```python
from build123d import *

# Parameters (mm, degrees)
F1_DEPTH  = 3.3
F0_W      = 178
F0_H      = 101.8
F2_DEPTH  = 2.5
F3_W      = 142.8
F3_H      = 4
F4_DEPTH  = 4
F5_R      = 1.99999
F7_D      = 2
F3_W_2    = 26.3
F8_DEPTH  = 0.1
F10_DEPTH = 0.5
F3_W_3    = 2.5
F3_H_2    = 8
F11_DEPTH = 10
F12_R     = 3.99999
F13_R     = 2
F14_DEPTH = 10


# Not quite as in the source:
# - a fillet or chamfer is up to 0.001 mm smaller than in the source, because OpenCascade refuses the exact size


with BuildPart() as f1:
    # F0 (on Front) → F1 (new body)
    with BuildSketch(Plane.XZ):
        with BuildLine():
            ThreePointArc((-75.5207621713, 74.1601898761), (-81.9271496089, 71.5065773137), (-84.5807621713, 65.1001898761))
            Line((-84.5807621713, 65.1001898761), (-84.5807621713, -35.3734344864))
            Line((-84.5807621713, -35.3734344864), (-84.5807621713, -55.8398101239))
            Line((-84.5807621713, -55.8398101239), (110.8192378287, -55.8398101239))
            Line((110.8192378287, -55.8398101239), (110.8192378287, -35.3734344864))
            Line((110.8192378287, -35.3734344864), (110.8192378287, 65.1001898761))
            ThreePointArc((110.8192378287, 65.1001898761), (108.1656252662, 71.5065773137), (101.7592378287, 74.1601898761))
            Line((101.7592378287, 74.1601898761), (-75.5207621713, 74.1601898761))
        make_face()
        with BuildLine():
            ThreePointArc((-83.3807621713, 65.1001898761), (-81.0786214714, 70.6580491763), (-75.5207621713, 72.9601898761))
            Line((-75.5207621713, 72.9601898761), (101.7592378287, 72.9601898761))
            ThreePointArc((101.7592378287, 72.9601898761), (107.3170971288, 70.6580491763), (109.6192378287, 65.1001898761))
            Line((109.6192378287, 65.1001898761), (109.6192378287, -29.9798101239))
            ThreePointArc((109.6192378287, -29.9798101239), (107.3170971288, -35.537669424), (101.7592378287, -37.8398101239))
            Line((101.7592378287, -37.8398101239), (-75.5207621713, -37.8398101239))
            ThreePointArc((-75.5207621713, -37.8398101239), (-81.0786214714, -35.537669424), (-83.3807621713, -29.9798101239))
            Line((-83.3807621713, -29.9798101239), (-83.3807621713, 65.1001898761))
        make_face(mode=Mode.SUBTRACT)
    extrude(amount=F1_DEPTH)

    # F0 (on Front) → F2 (join)
    with BuildSketch(Plane.XZ):
        with BuildLine():
            Line((101.7592378287, 72.9601898761), (-75.5207621713, 72.9601898761))
            ThreePointArc((-75.5207621713, 72.9601898761), (-81.0786214714, 70.6580491763), (-83.3807621713, 65.1001898761))
            Line((-83.3807621713, 65.1001898761), (-83.3807621713, -29.9798101239))
            ThreePointArc((-83.3807621713, -29.9798101239), (-81.0786214714, -35.537669424), (-75.5207621713, -37.8398101239))
            Line((-75.5207621713, -37.8398101239), (101.7592378287, -37.8398101239))
            ThreePointArc((101.7592378287, -37.8398101239), (107.3170971288, -35.537669424), (109.6192378287, -29.9798101239))
            Line((109.6192378287, -29.9798101239), (109.6192378287, 65.1001898761))
            ThreePointArc((109.6192378287, 65.1001898761), (107.3170971288, 70.6580491763), (101.7592378287, 72.9601898761))
        make_face()
        with Locations((9.6192378287, 16.0601898761)):
            Rectangle(F0_W, F0_H, mode=Mode.SUBTRACT)
    extrude(amount=F2_DEPTH)

    # F3 (on face) → F4 (join)
    with BuildSketch(Plane(origin=(0, 0, 0), x_dir=(-1, 0, 0), z_dir=(0, 1, 0))):
        with Locations((-13.1192378287, -53.8398101239)):
            Rectangle(F3_W, F3_H)
    extrude(amount=F4_DEPTH)

    # F5 (radius 2 in the source; OpenCascade refuses exactly that, so slightly less here)
    f5_edges = [f1.edges().sort_by_distance(p)[0] for p in [
        (13.119238, 4, -51.83981),
        (13.119238, 4, -55.83981),
    ]]
    fillet(f5_edges, radius=F5_R)

    # F7 (through all)
    with Locations(Plane.YZ.offset(84.5192378287)):
        with Locations((2, -53.8398101239)):
            Hole(F7_D / 2)

    # F3 (on face) → F8 (cut)
    with BuildSketch(Plane(origin=(0, 0, 0), x_dir=(-1, 0, 0), z_dir=(0, 1, 0))):
        with Locations((-97.6692378287, -53.8398101239)):
            Rectangle(F3_W_2, F3_H)
        with Locations((71.4307621713, -53.8398101239)):
            Rectangle(F3_W_2, F3_H)
    extrude(amount=-F8_DEPTH, mode=Mode.SUBTRACT)

    # F9 (on face) → F10 (join)
    with BuildSketch(Plane.XZ.offset(3.3)):
        with BuildLine():
            Line((101.7592378287, 74.1601898761), (-75.5207621713, 74.1601898761))
            ThreePointArc((-75.5207621713, 74.1601898761), (-81.9271496089, 71.5065773137), (-84.5807621713, 65.1001898761))
            Line((-84.5807621713, 65.1001898761), (-84.5807621713, -55.8398101239))
            Line((-84.5807621713, -55.8398101239), (110.8192378287, -55.8398101239))
            Line((110.8192378287, -55.8398101239), (110.8192378287, 65.1001898761))
            ThreePointArc((110.8192378287, 65.1001898761), (108.1656252662, 71.5065773137), (101.7592378287, 74.1601898761))
        make_face()
        with BuildLine():
            add(Edge.make_bspline(
                [(14.902347951, -49.9172276662), (15.0190761779, -50.0441554468), (15.2457329289, -50.0441554468)],
                knots=[0, 0, 0, 1, 1, 1], degree=2))
            add(Edge.make_bspline(
                [(15.2457329289, -50.0441554468), (15.5585192454, -50.0441554468), (15.8418401843, -49.9308270713)],
                knots=[0, 0, 0, 1, 1, 1], degree=2))
            Line((15.8418401843, -49.9308270713), (15.8418401843, -50.8737191558))
            add(Edge.make_bspline(
                [(15.8418401843, -50.8737191558), (15.3454618994, -51.016512909), (14.8989480998, -51.016512909)],
                knots=[0, 0, 0, 1, 1, 1], degree=2))
            add(Edge.make_bspline(
                [(14.8989480998, -51.016512909), (14.2552429267, -51.016512909), (13.9186576513, -50.6867273361)],
                knots=[0, 0, 0, 1, 1, 1], degree=2))
            add(Edge.make_bspline(
                [(13.9186576513, -50.6867273361), (13.582072376, -50.3569417633), (13.582072376, -49.7835001831)],
                knots=[0, 0, 0, 1, 1, 1], degree=2))
            add(Edge.make_bspline(
                [(13.582072376, -49.7835001831), (13.582072376, -49.3505857885), (13.7090001566, -48.7703445057)],
                knots=[0, 0, 0, 1, 1, 1], degree=2))
            Line((13.7090001566, -48.7703445057), (14.6654916462, -44.144280216))
            Line((14.6654916462, -44.144280216), (11.8662807702, -44.144280216))
            Line((11.8662807702, -44.144280216), (10.4156775633, -50.8737191558))
            Line((10.4156775633, -50.8737191558), (9.212130215, -50.8737191558))
            Line((9.212130215, -50.8737191558), (10.662733422, -44.144280216))
            Line((10.662733422, -44.144280216), (9.0988018395, -44.144280216))
            Line((9.0988018395, -44.144280216), (9.1826648374, -43.6773673088))
            Line((9.1826648374, -43.6773673088), (10.5788704241, -43.1107254311))
            Line((10.5788704241, -43.1107254311), (17.5553652225, -43.1107254311))
            Line((17.5553652225, -43.1107254311), (17.335508174, -44.144280216))
            Line((17.335508174, -44.144280216), (15.8554395894, -44.144280216))
            Line((15.8554395894, -44.144280216), (14.8694827221, -48.8836728813))
            add(Edge.make_bspline(
                [(14.8694827221, -48.8836728813), (14.7856197242, -49.2939216007), (14.7856197242, -49.5840422421)],
                knots=[0, 0, 0, 1, 1, 1], degree=2))
            add(Edge.make_bspline(
                [(14.7856197242, -49.5840422421), (14.7856197242, -49.7902998856), (14.902347951, -49.9172276662)],
                knots=[0, 0, 0, 1, 1, 1], degree=2))
        make_face(mode=Mode.SUBTRACT)
        with BuildLine():
            Line((-83.3807621713, -29.9798101239), (-83.3807621713, 65.1001898761))
            ThreePointArc((-83.3807621713, 65.1001898761), (-81.0786214714, 70.6580491763), (-75.5207621713, 72.9601898761))
            Line((-75.5207621713, 72.9601898761), (101.7592378287, 72.9601898761))
            ThreePointArc((101.7592378287, 72.9601898761), (107.3170971288, 70.6580491763), (109.6192378287, 65.1001898761))
            Line((109.6192378287, 65.1001898761), (109.6192378287, -29.9798101239))
            ThreePointArc((109.6192378287, -29.9798101239), (107.3170971288, -35.537669424), (101.7592378287, -37.8398101239))
            Line((101.7592378287, -37.8398101239), (-75.5207621713, -37.8398101239))
            ThreePointArc((-75.5207621713, -37.8398101239), (-81.0786214714, -35.537669424), (-83.3807621713, -29.9798101239))
        make_face(mode=Mode.SUBTRACT)
    extrude(amount=F10_DEPTH)

    # F3 (on face) → F11 (join)
    with BuildSketch(Plane(origin=(0, 0, 0), x_dir=(-1, 0, 0), z_dir=(0, 1, 0))):
        with Locations((-109.0692378287, -22.8345717341)):
            Rectangle(F3_W_3, F3_H_2)
        with Locations((-104.1692378287, -22.8345717341)):
            Rectangle(F3_W_3, F3_H_2)
    extrude(amount=F11_DEPTH)

    # F12 (radius 4 in the source; OpenCascade refuses exactly that, so slightly less here)
    f12_edges = [f1.edges().sort_by_distance(p)[0] for p in [
        (109.069238, 10, -18.834572),
        (109.069238, 10, -26.834572),
        (104.169238, 10, -18.834572),
        (104.169238, 10, -26.834572),
    ]]
    fillet(f12_edges, radius=F12_R)

    # F13 (on face) → F14 (cut)
    with BuildSketch(Plane.YZ.offset(110.3192378287)):
        with Locations((6, -22.8345717341)):
            Circle(F13_R)
    extrude(amount=-F14_DEPTH, mode=Mode.SUBTRACT)


solid = f1.part
```
The model under review builds one solid part; all positions refer to its coordinate system, in mm. A direction names the side the tool comes from. Coordinates: 2 decimals unless noted, no trailing zeros. Loops run counter-clockwise (first coordinate to the right, second up) from the corner with the lowest first, then second, coordinate; pieces in that order, holes last. Notation, with made-up numbers: (63, -12.5) -> (82, -12.5) arc R20 ccw to (82, 12.5) -> close; hole circle Ø10 at (-19, 0). An arc over 180 degrees is marked (long way). Answer as CSV lines item,"result".
Item 1: Take a section at A-A, the plane z = 11. State the section outline as (x, y) points, and give its area (3 significant figures).
Results below:
outline,"(-84.58, -3.8) -> (-83.38, -3.8) -> (-83.38, -2.5) -> (-79.38, -2.5) -> (-79.38, 0) -> (-84.58, 0) -> close; (98.62, -2.5) -> (109.62, -2.5) -> (109.62, -3.8) -> (110.82, -3.8) -> (110.82, 0) -> (98.62, 0) -> close"
area,"46.6 mm2"
Item 2: Machinability: for faces 1 (the cylindrical face through (109.05, 8.8, -19.98)), 2 (the cylindrical face through (109.05, 8.8, -25.69)), 3 (the flat face through (98, -0.1, -54)), 4 (the cylindrical face through (-81.139, -3.141, 70.597)), which of the approach directions +Z, -Z, +X, -X, +Y, -Y give a long, thin tool a straight path to every point of the face, cutting with its end or side? Answer none if there is none.
Results below:
face 1,"+Z, +X, -X, +Y"
face 2,"-Z, +X, -X, +Y"
face 3,"-Z, +X, +Y"
face 4,"-Y"
Item 3: Insertion check: pin 1 (4.5 mm diameter, centred on x = -70, z = -53.5, fed in from +Y); pin 2 (4 mm diameter, centred on y = 3.5, z = -23, fed in from -X); pin 3 (3 mm diameter, centred on x = 104, y = 3, fed in from -Z). Each pin has a flat end and moves straight along its axis. Give the tip position at first contact, or say it passes through.
Results below:
pin 1,"stops at y = 0"
pin 2,"stops at x = 102.92"
pin 3,"stops at z = -26.83"
Item 4: Draft analysis for pull direction X (two halves, no side actions). For faces 5 (the flat face through (-84.581, -2, 5)), 6 (the flat face through (110.319, 3.8, -22.9)), 7 (the flat face through (107.819, 3.8, -22.9)), 8 (the cylindrical face through (109.09, 4.53, -21.48)), state which applies: +X half, -X half, draft (parallel to the pull), parting line (faces both ways), or undercut.
Results below:
face 5,"-X half"
face 6,"+X half"
face 7,"undercut"
face 8,"draft"
Item 5: For L1, parallel to Z at x = 40.5, y = 2; L2, parallel to Z at x = 31.5, y = -3; L3, parallel to X at y = -1.5, z = 26, list the stretches that pass through material, from the lowest coordinate up.
Results below:
L1,"z = -55.84 to -54.84, -52.84 to -51.84"
L2,"z = -55.84 to -37.84, 72.96 to 74.16"
L3,"x = -84.58 to -79.38, 98.62 to 110.82"
Item 6: Take a section at B-B, the plane x = -3. Count the separate pieces of the cut face and the enclosed holes in it, and give its area (3 significant figures).
Results below:
separate pieces,"2"
enclosed holes,"1"
area,"107 mm2"
